```python
from build123d import *

# Parameters (mm, degrees)
F0_W     = 152.4
F0_H     = 177.8
F0_R     = 1.8415
F0_R_2   = 1.85447
F0_R_3   = 3.942651
F0_R_4   = 1.873541
F1_DEPTH = 6.35


with BuildPart() as f1:
    # F0 (on Front) → F1 (new body)
    with BuildSketch(Plane.XZ):
        Rectangle(F0_W, F0_H)
        with Locations((-16.722151, -9.654538)):
            Circle(F0_R, mode=Mode.SUBTRACT)
        with Locations((16.717754, -9.652)):
            Circle(F0_R_2, mode=Mode.SUBTRACT)
        Circle(F0_R_3, mode=Mode.SUBTRACT)
        with Locations((0, 19.304)):
            Circle(F0_R_4, mode=Mode.SUBTRACT)
    extrude(amount=F1_DEPTH)


solid = f1.part
```
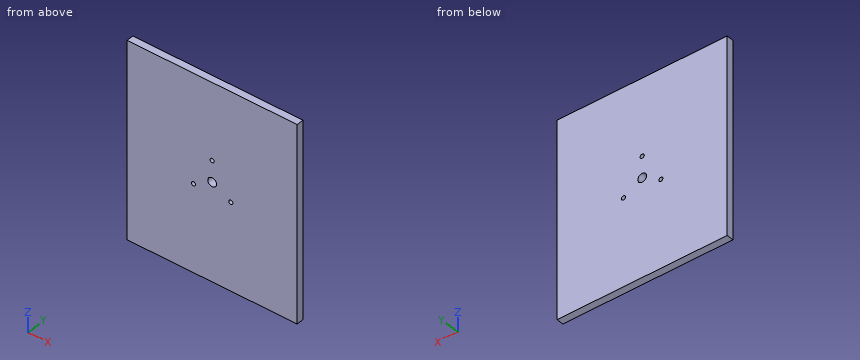
CAD build for the part. Positions are in the model's coordinates, mm. Give positions to 0.01 mm unless a question says otherwise; leave off trailing zeros. Write each loop counter-clockwise with the first axis right and the second up, starting at its lowest first coordinate (ties: lowest second). Pieces come first, ordered by that corner, then holes. Notation, with made-up numbers: (28.5, 85.25) -> (32.5, 85.25) arc R23 cw to (32.5, 112.25) -> close; hole circle Ø3 at (65, 74). An arc over 180 degrees is marked (long way). Write each question's results on one line, items separated by ' | '.
1. Cut at A-A, the plane z = 0. Write the cut outline in (x, y), then the cut area to 3 significant figures.
Geometry check:
outline: (-76.2, -6.35) -> (-3.94, -6.35) -> (-3.94, 0) -> (-76.2, 0) -> close; (3.94, -6.35) -> (76.2, -6.35) -> (76.2, 0) -> (3.94, 0) -> close | area: 918 mm²
2. Wall check: probe 1 along X at (y, z) = (-5.75, 19.5); probe 2 along Z at (x, y) = (0, -4.5); probe 3 along Z at (x, y) = (17, -1). Give the ranges that are in metal, low to high. Write a range as [from, to].
Geometry check:
probe 1: [-76.2, -1.86], [1.86, 76.2] | probe 2: [-88.9, -3.94], [3.94, 17.43], [21.18, 88.9] | probe 3: [-88.9, -11.48], [-7.82, 88.9]
3. Drop a flat-ended pin along its axis: P1, Ø6, axis at x = -16.72, z = -9.65, coming from the +Y side. Give the stop position or say it passes through.
Geometry check:
P1: y = 0
